from build123d import *

# Parameters (mm, degrees)
F1_DEPTH    = 12.7
F2_R        = 3.175
F2_R_2      = 2.5796875
F3_DEPTH    = 14.2885
F2_R_3      = 4.7625
F4_DEPTH    = 4.7625
F7_T1_DEPTH = 23.7232420224
F7_T3_DEPTH = 21.5242768354
F8_W        = 32.2767272592
F8_H        = 15.9856376707
F9_DEPTH    = 1.905


# Not quite as in the source:
# - a fillet or chamfer that OpenCascade refuses, or shapes differently, is made with other operations: its cross-section is extruded or revolved along the edge and cut away or added


with BuildPart() as f1:
    # F0 (on Front) → F1 (new body)
    with BuildSketch(Plane.XZ):
        with BuildLine():
            ThreePointArc((-35.0237072996, 5.55625), (-22.5238733613, 10.7338507446), (-14.2875, 0))
            Line((-14.2875, 0), (0, 0))
            Line((0, 0), (14.2875, 0))
            ThreePointArc((14.2875, 0), (22.5238733613, 10.7338507446), (35.0237072996, 5.55625))
            Line((35.0237072996, 5.55625), (37.7733379566, 7.14375))
            ThreePointArc((37.7733379566, 7.14375), (32.54375, 12.3733379566), (25.4, 14.2875))
            Line((25.4, 14.2875), (0, 14.2875))
            Line((0, 14.2875), (-25.4, 14.2875))
            ThreePointArc((-25.4, 14.2875), (-32.54375, 12.3733379566), (-37.7733379566, 7.14375))
            Line((-37.7733379566, 7.14375), (-35.0237072996, 5.55625))
        make_face()
    extrude(amount=F1_DEPTH)

    # F2 (on face) → F3 (cut, through all)
    with BuildSketch(Plane.XY.offset(14.2875)):
        with Locations((9.525, -6.35)):
            Circle(F2_R)
        with Locations((-9.525, -6.35)):
            Circle(F2_R_2)
    extrude(amount=-F3_DEPTH, mode=Mode.SUBTRACT)

    # F2 (on face) → F4 (cut)
    with BuildSketch(Plane.XY.offset(14.2875)):
        with Locations((9.525, -6.35)):
            Circle(F2_R_3)
        with Locations((9.525, -6.35)):
            Circle(F2_R, mode=Mode.SUBTRACT)
    extrude(amount=-F4_DEPTH, mode=Mode.SUBTRACT)

    # F7: fillet of radius 1.905 on 4 edges, made by hand

    # F7_s2 → F7_t1 (cut)
    with BuildSketch(Plane.XZ.offset(-5.5116210112)):
        with BuildLine():
            ThreePointArc((-35.9958935884, 6.1175420156), (-36.9160377964, 7.4177082385), (-36.526992602, 8.9622927805))
            ThreePointArc((-36.526992602, 8.9622927805), (-37.1852941649, 8.0770971084), (-37.7733379566, 7.14375))
            Line((-37.7733379566, 7.14375), (-35.9958935884, 6.1175420156))
        make_face()
        with BuildLine():
            ThreePointArc((35.9958935884, 6.1175420156), (36.9160377964, 7.4177082385), (36.526992602, 8.9622927805))
            ThreePointArc((36.526992602, 8.9622927805), (37.1852941649, 8.0770971084), (37.7733379566, 7.14375))
            Line((37.7733379566, 7.14375), (35.9958935884, 6.1175420156))
        make_face()
    extrude(amount=F7_T1_DEPTH, mode=Mode.SUBTRACT)

    # F7_s4 → F7_t3 (cut)
    with BuildSketch(Plane.XZ.offset(-4.4121384177)):
        with BuildLine():
            ThreePointArc((-34.1069900207, 6.9047795786), (-35.242899906, 6.2171522544), (-36.5521168814, 6.4386776835))
            Line((-36.5521168814, 6.4386776835), (-35.0237072996, 5.55625))
            ThreePointArc((-35.0237072996, 5.55625), (-34.5901169235, 6.2473520136), (-34.1069900207, 6.9047795786))
        make_face()
        with BuildLine():
            ThreePointArc((34.1069900207, 6.9047795786), (35.242899906, 6.2171522544), (36.5521168814, 6.4386776835))
            Line((36.5521168814, 6.4386776835), (35.0237072996, 5.55625))
            ThreePointArc((35.0237072996, 5.55625), (34.5901169235, 6.2473520136), (34.1069900207, 6.9047795786))
        make_face()
    extrude(amount=F7_T3_DEPTH, mode=Mode.SUBTRACT)

    # F8 (on face) → F9 (cut)
    with BuildSketch(Plane(origin=(0, 0, 0), x_dir=(1, 0, 0), z_dir=(0, 0, -1))):
        with Locations((0, 6.0593477681)):
            Rectangle(F8_W, F8_H)
    extrude(amount=-F9_DEPTH, mode=Mode.SUBTRACT)


solid = f1.part
Can you work these out from the model? Positions are in its coordinate system, mm. A direction names the side the tool comes from. Give positions to 0.01 mm unless a question says otherwise; leave off trailing zeros. Order: outer loops, then holes, each group sorted by start corner. A loop starts at its lowest first (then second) coordinate and runs counter-clockwise, first axis right, second up. Notation, with made-up numbers: M 78,86.25 L 107,86.25 A23 ccw 107,102.25 Z; hole C 79,-32 d8. An arc over 180 degrees is marked long. Use a Markdown table: item, result. Add a question column.
Item 1: If I drill on L1, parallel to X at y = -7, z = 11.75; L2, parallel to X at y = -4.75, z = 4; L3, parallel to Z at x = -25, y = -4.25, over which ranges is the centre line in solid material (lowest first)? Write a range as [from, to].
Item 2: Suppose I cut it at A-A (y = -6.35). Count the separate pieces of the cut face and the enclosed holes in it, then the cut area to 3 significant figures.
Item 3: Suppose I cut it at B-B (z = 8.25). List the corners of the cut face in (x, y) for me (3 decimals).
Item 4: Suppose I cut it at C-C (x = -8). List the corners of the cut face in (y, z) for me (1 decimal).
Item 5: We'd pull the mould along Y, two halves only. Please class faces 1 (the cylindrical face through (-22.83, -6.26, 10.81)), 2 (the flat face through (-1, -12.7, 10)), 3 (the flat face through (13, -7, 9.525)), 4 (the flat face through (-1, 0, 10)): +Y half, -Y half, draft (parallel to the pull), parting line (faces both ways), or undercut.
Item 6: For faces 5 (the cylindrical face through (12.085, -2.334, 11.94)), 6 (the cylindrical face through (35.07, -6.26, 6.26)), which set-ups out of +Z, -Z, +X, -X, +Y, -Y let a thin tool reach every point of the face, with its end or its side?
Item 7: Will these pins go through, and if not, where does the flat tip stop? pin 1 (1.5 mm diameter, centred on x = 20, y = -8, fed in from -Z); pin 2 (5 mm diameter, centred on y = -10, z = 10.5, fed in from +X); pin 3 (6 mm diameter, centred on y = -11.5, z = 4, fed in from +X).
Item 8: Suppose I cut it at D-D (z = 3). List the corners of the cut face in (x, y) for me (3 decimals), then the cut area to 3 significant figures.
Answer sheet:
| question | item | result |
|---|---|---|
| 1 | L1 | x = [-33.53, -12.02], [-7.03, 4.81], [14.24, 33.53] |
| 1 | L2 | x = [-15.03, -11.55], [-7.5, 6.78], [12.27, 15.03] |
| 1 | L3 | z = [11.11, 14.29] |
| 2 | separate pieces | 3 |
| 2 | enclosed holes | 0 |
| 2 | area | 401 mm² |
| 3 | outline | M -36.886,-12.7 L -32.845,-12.7 L -32.845,0 L -36.886,0 Z; M -17.955,-12.7 L 17.955,-12.7 L 17.955,0 L -17.955,0 Z; M 32.845,-12.7 L 36.886,-12.7 L 36.886,0 L 32.845,0 Z; hole C -9.525,-6.35 d5.159; hole C 9.525,-6.35 d6.35 |
| 4 | outline | M -12.7,1.9 L -8.4,1.9 L -8.4,14.3 L -12.7,14.3 Z; M -4.3,1.9 L 0,1.9 L 0,14.3 L -4.3,14.3 Z |
| 5 | face 1 | draft |
| 5 | face 2 | -Y half |
| 5 | face 3 | undercut |
| 5 | face 4 | +Y half |
| 6 | face 5 | +Z |
| 6 | face 6 | -Z, +Y, -Y |
| 7 | pin 1 | stops at z = 9.26 |
| 7 | pin 2 | stops at x = 36.93 |
| 7 | pin 3 | stops at x = 36.79 |
| 8 | outline | M -14.7,-12.7 L 14.7,-12.7 L 14.7,0 L -14.7,0 Z; hole C -9.525,-6.35 d5.159; hole C 9.525,-6.35 d6.35 |
| 8 | area | 321 mm² |
